Geometry: final body of the model. Coordinates: model frame, mm. Face numbers are marked on the shaded views. A direction names the side the tool comes from. Coordinates: 2 decimals unless noted, no trailing zeros. Write each loop counter-clockwise with the first axis right and the second up, starting at its lowest first coordinate (ties: lowest second). Pieces come first, ordered by that corner, then holes.
from build123d import *

# Parameters (mm, degrees)
F2_SIZE = 6


with BuildPart() as f1:
    # F0 (on Front) → F1 (revolve)
    with BuildSketch(Plane.XZ):
        with BuildLine():
            ThreePointArc((-103.6, 102.320508), (-108.423619, 104.318517), (-113.6, 105))
            Line((-113.6, 105), (-150, 105))
            Line((-150, 105), (-150, 93.55))
            Line((-150, 93.55), (-130, 93.55))
            Line((-130, 93.55), (-50, 30))
            Line((-50, 30), (-10, 30))
            ThreePointArc((-10, 30), (-3.532095, 32.373323), (-0.134275, 38.366759))
            ThreePointArc((-0.134275, 38.366759), (-1.778554, 42.426305), (-5, 45.393772))
            Line((-5, 45.393772), (-103.6, 102.320508))
        make_face()
    revolve(axis=Axis((-75, 0, 0), (-1, 0, 0)))

    # F2
    f2_edges = [f1.edges().sort_by_distance(p)[0] for p in [
        (-150, 0, -105),
    ]]
    chamfer(f2_edges, length=F2_SIZE)


solid = f1.part
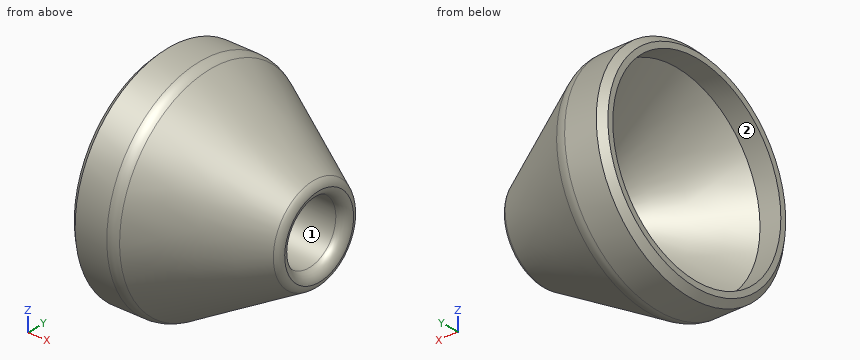
Item 1: Pin query (flat end, axial travel): pin 1 (12 mm diameter, centred on x = -42, y = -21.5, fed in from -Z); pin 2 (1.5 mm diameter, centred on x = -92.5, z = 23.5, fed in from -Y); pin 3 (5 mm diameter, centred on x = -48.5, z = -61.5, fed in from +Y) (3 decimals). Return the tip coordinate at first contact, or that it passes through.
Derived:
pin 1: stops at z = -67.27
pin 2: stops at y = -93.47
pin 3: stops at y = 39.425
Item 2: Set-up query: the marked faces 1 and 2. Return all of +Z, -Z, +X, -X, +Y, -Y with unobstructed straight access to the full face (end or side cutting, diameter ignored); none if empty.
Derived:
face 1: +X, -X
face 2: -X
Item 3: Section D-D, the plane x = -14. Output: boundary loops of the cut face in (y, z).
Derived:
outline: circle Ø101.18 at (0, 0); hole circle Ø60 at (0, 0)
Item 4: Section A-A, the plane z = 0. Output: boundary loops of the cut face in (x, y), plus the area to 3 significant figures.
Derived:
outline: (-150, -99) - (-144, -105) - (-113.6, -105) arc R20 ccw to (-103.6, -102.32) - (-5, -45.39) arc R10 ccw to (-0.13, -38.37) arc R10 ccw to (-10, -30) - (-50, -30) - (-130, -93.55) - (-150, -93.55) - close; (-150, 93.55) - (-130, 93.55) - (-50, 30) - (-10, 30) arc R10 ccw to (-0.13, 38.37) arc R10 ccw to (-5, 45.39) - (-103.6, 102.32) arc R20 ccw to (-113.6, 105) - (-144, 105) - (-150, 99) - close
area: 8,020 mm2
Item 5: Section C-C, the plane x = -80.5. Output: boundary loops of the cut face in (y, z).
Derived:
outline: circle Ø177.97 at (0, 0); hole circle Ø108.46 at (0, 0)
Item 6: Material intervals for probe 1 along Y at (x, z) = (-139.25, 0); probe 2 along Z at (x, y) = (-98, 44); probe 3 along Y at (x, z) = (-73, 2), sorted ascending.
Derived:
probe 1: y = -105 to -93.55, 93.55 to 105
probe 2: z = -88.78 to -52.02, 52.02 to 88.78
probe 3: y = -84.63 to -48.23, 48.23 to 84.63
